Geometry check sheet. Reference: the model listing, model coordinates, mm. A direction names the side the tool comes from. Round coordinates to 2 decimals unless told otherwise and drop trailing zeros. Order: outer loops, then holes, each group sorted by start corner. A loop starts at its lowest first (then second) coordinate and runs counter-clockwise, first axis right, second up. Notation, with made-up numbers: (-12.5, 11) - (34.5, 11) arc R10 cw to (34.5, 19) - close; hole circle Ø6 at (60, -2.5). An arc over 180 degrees is marked (long way). Return JSON: item names as keys, results as strings. Group by question number.
Q1. Sectioned sample at C-C, the plane z = 14. Record the cut outline in (x, y).
Q2. Draft check along Z on faces 1 (the flat face through (15, -5, 10)), 2 (the cylindrical face through (10.616, -5.208, 15.586)), 3 (the flat face through (7, -5, 0)), 4 (the cylindrical face through (14.442, -5.208, 15.586)). Enter one of: pulls with the +Z half, pulls with the -Z half, needs draft (parallel to the pull), parting line crosses it, or undercut.
Q3. Sectioned sample at B-B, the plane x = 5. Record the cut outline in (y, z) (3 decimals), then the cut area to 4 significant figures.
Q4. Material ranges on line 1 along X through (y, z) = (-7.5, 14); line 2 along Y through (x, z) = (10.4, 14); line 3 along Z through (x, y) = (10.45, -5), recorded low to high.
Q5. Sectioned sample at D-D, the plane x = 12.25. Record the cut outline in (y, z).
Q6. Gauge pin test, flat ends, axial feed: pin 1 Ø1.9 at (y, z) = (-5, 14) entering from +X; pin 2 Ø5 at (x, y) = (3.5, -3.5) entering from +Z; pin 3 Ø3 at (y, z) = (-5.5, 15) entering from -X; pin 4 Ø0.8 at (x, z) = (12, 16) entering from +Y. Record the tip position at first contact, or that the pin passes through.
Q7. Tool access check on faces 5 (the flat face through (12.56, -6.49, 11.46)), 6 (the flat face through (10, -3.8, 12.6)), 7 (the flat face through (14.2, -4.9, 20)). Record the directions out of +Z, -Z, +X, -X, +Y, -Y that give a thin tool (end or side, any length) a straight path to the whole face; none if there is none.
Q8. Sectioned sample at A-A, the plane z = 16.75. Record the cut outline in (x, y).
```python
from build123d import *

# Parameters (mm, degrees)
PAD_DEPTH       = 10
SKETCH001_R     = 1.6
POCKET_DEPTH    = 20.001
SKETCH002_R     = 1.6
POCKET001_DEPTH = 15.001
POCKET002_DEPTH = 2.65
SKETCH004_R     = 3.125
POCKET003_DEPTH = 3


with BuildPart() as part:
    # Sketch → Pad (new body)
    with BuildSketch(Plane.XZ):
        Polygon((15, 20), (10, 20), (10, 5), (0, 5), (0, 0), (15, 0), (15, 14), align=None)
    extrude(amount=PAD_DEPTH)

    # Sketch001 → Pocket (cut, through all)
    with BuildSketch(Plane.XY):
        with Locations((5, -5)):
            Circle(SKETCH001_R)
    extrude(amount=POCKET_DEPTH, mode=Mode.SUBTRACT)

    # Sketch002 → Pocket001 (cut, through all)
    with BuildSketch(Plane.YZ):
        with Locations((-5, 14)):
            Circle(SKETCH002_R)
    extrude(amount=POCKET001_DEPTH, mode=Mode.SUBTRACT)

    # Sketch003 → Pocket002 (cut)
    with BuildSketch(Plane.YZ.offset(11.25)):
        Polygon((-2.055514, 12.3), (-2.055514, 15.7), (-2.055514, 20.7), (-7.944486, 20.7), (-7.944486, 15.7), (-7.944486, 12.3), (-5, 10.6), align=None)
    extrude(amount=POCKET002_DEPTH, mode=Mode.SUBTRACT)

    # Sketch004 → Pocket003 (cut)
    with BuildSketch(Plane.XY.offset(5)):
        with Locations((5, -5)):
            Circle(SKETCH004_R)
    extrude(amount=-POCKET003_DEPTH, mode=Mode.SUBTRACT)


solid = part.part
```
Reply:
{
 "1": {"outline": "(10, -10) - (15, -10) - (15, -6.6) - (13.9, -6.6) - (13.9, -7.94) - (11.25, -7.94) - (11.25, -6.6) - (10, -6.6) - close; (10, -3.4) - (11.25, -3.4) - (11.25, -2.06) - (13.9, -2.06) - (13.9, -3.4) - (15, -3.4) - (15, 0) - (10, 0) - close"},
 "2": {"face 1": "needs draft", "face 2": "undercut", "face 3": "pulls with the -Z half", "face 4": "undercut"},
 "3": {"outline": "(-10, 0) - (-6.6, 0) - (-6.6, 2) - (-8.125, 2) - (-8.125, 5) - (-10, 5) - close; (-3.4, 0) - (0, 0) - (0, 5) - (-1.875, 5) - (-1.875, 2) - (-3.4, 2) - close", "area": "24.85 mm^2"},
 "4": {"line 1": "10 to 11.25, 13.9 to 15", "line 2": "-10 to -6.6, -3.4 to 0", "line 3": "0 to 12.4, 15.6 to 20"},
 "5": {"outline": "(-10, 0) - (0, 0) - (0, 20) - (-2.06, 20) - (-2.06, 12.3) - (-5, 10.6) - (-7.94, 12.3) - (-7.94, 20) - (-10, 20) - close"},
 "6": {"pin 1": "through", "pin 2": "z = 5", "pin 3": "x = 10", "pin 4": "y = 0"},
 "7": {"face 5": "+Z", "face 6": "+Z, -X, +Y, -Y", "face 7": "+Z, +X, -X, +Y, -Y"},
 "8": {"outline": "(10, -10) - (15, -10) - (15, 0) - (10, 0) - close; hole (11.25, -7.94) - (13.9, -7.94) - (13.9, -2.06) - (11.25, -2.06) - close"}
}
